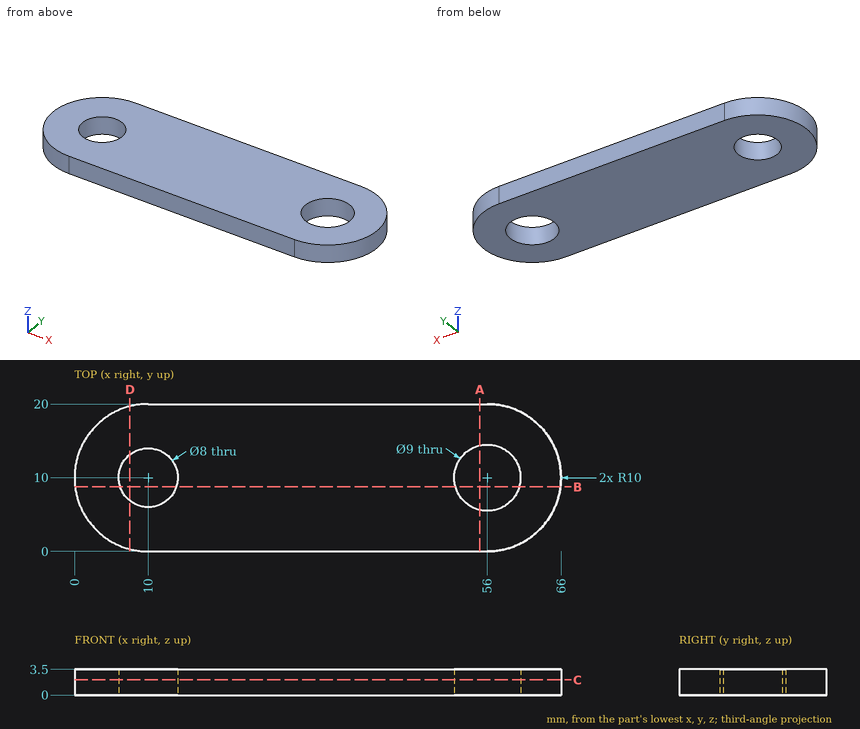
Input: dimensioned drawing with shaded views. Units: mm. Origin: part minimum x, y, z. Round coordinates to 2 decimals unless told otherwise and drop trailing zeros. Loops run counter-clockwise (first coordinate to the right, second up) from the corner with the lowest first, then second, coordinate; pieces in that order, holes last. Notation, with made-up numbers: M 51,51 L 76,51 A16 ccw 76,59 Z; hole C 0,32 d7. An arc over 180 degrees is marked long. One line per question, with ' | ' between items.
(1) Contact query for flat-ended pins moving along their axis: P1, Ø2, axis at y = 11.5, z = 1.5, coming from the -X side; P2, Ø2, axis at y = 13, z = 2.5, coming from the +X side; P3, Ø5, axis at x = 10, y = 10, coming from the +Z side; P4, Ø1.5, axis at y = 16, z = 3, coming from the -X side. Output: stop coordinate, or through.
Check result:
P1: stops at x = 0.01 | P2: stops at x = 65.8 | P3: passes through | P4: stops at x = 1.49
(2) Cut plane C-C on z = 2.1. Return the cut outline in (x, y).
Check result:
outline: M 10,0 L 56,0 A10 ccw 56,20 L 10,20 A10 ccw Z; hole C 10,10 d8; hole C 56,10 d9
(3) Cut plane B-B on y = 8.75. Return the cut outline in (x, z), plus the area to 3 significant figures.
Check result:
outline: M 0.08,0 L 6.2,0 L 6.2,3.5 L 0.08,3.5 Z; M 13.8,0 L 51.68,0 L 51.68,3.5 L 13.8,3.5 Z; M 60.32,0 L 65.92,0 L 65.92,3.5 L 60.32,3.5 Z | area: 174 mm2
(4) Material intervals for line 1 along X through (y, z) = (10, 2); line 2 along Y through (x, z) = (56, 1.05); line 3 along Y through (x, z) = (10, 1.15), sorted ascending. Write a range as from..to.
Check result:
line 1: x = 0..6, 14..51.5, 60.5..66 | line 2: y = 0..5.5, 14.5..20 | line 3: y = 0..6, 14..20
(5) Cut plane A-A on x = 55. Return the cut outline in (y, z), plus the area to 3 significant figures.
Check result:
outline: M 0,0 L 5.61,0 L 5.61,3.5 L 0,3.5 Z; M 14.39,0 L 20,0 L 20,3.5 L 14.39,3.5 Z | area: 39.3 mm2
(6) Cut plane D-D on x = 7.5. Return the cut outline in (y, z), plus the area to 3 significant figures.
Check result:
outline: M 0.32,0 L 6.88,0 L 6.88,3.5 L 0.32,3.5 Z; M 13.12,0 L 19.68,0 L 19.68,3.5 L 13.12,3.5 Z | area: 45.9 mm2
